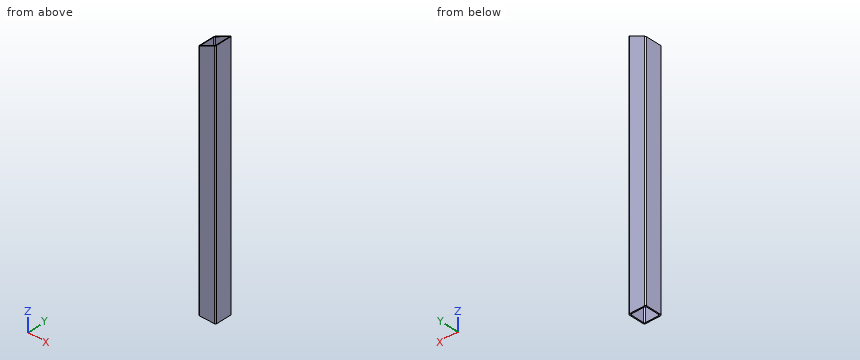
```python
from build123d import *

# Parameters (mm, degrees)
F1_DEPTH      = 723.9
F3_DEPTH      = 50.8
F3_DEPTH_BACK = 50.8


with BuildPart() as f1:
    # F0 (on Top) → F1 (new body)
    with BuildSketch(Plane.XY):
        with BuildLine():
            ThreePointArc((25.4, 22.225), (24.4700640303, 24.4700640303), (22.225, 25.4))
            Line((22.225, 25.4), (-22.225, 25.4))
            ThreePointArc((-22.225, 25.4), (-24.4700640303, 24.4700640303), (-25.4, 22.225))
            Line((-25.4, 22.225), (-25.4, -22.225))
            ThreePointArc((-25.4, -22.225), (-24.4700640303, -24.4700640303), (-22.225, -25.4))
            Line((-22.225, -25.4), (22.225, -25.4))
            ThreePointArc((22.225, -25.4), (24.4700640303, -24.4700640303), (25.4, -22.225))
            Line((25.4, -22.225), (25.4, 22.225))
        make_face()
        with BuildLine():
            Line((-19.05, 22.225), (19.05, 22.225))
            ThreePointArc((19.05, 22.225), (21.2950640303, 21.2950640303), (22.225, 19.05))
            Line((22.225, 19.05), (22.225, -19.05))
            ThreePointArc((22.225, -19.05), (21.2950640303, -21.2950640303), (19.05, -22.225))
            Line((19.05, -22.225), (-19.05, -22.225))
            ThreePointArc((-19.05, -22.225), (-21.2950640303, -21.2950640303), (-22.225, -19.05))
            Line((-22.225, -19.05), (-22.225, 19.05))
            ThreePointArc((-22.225, 19.05), (-21.2950640303, 21.2950640303), (-19.05, 22.225))
        make_face(mode=Mode.SUBTRACT)
    extrude(amount=F1_DEPTH)

    # F2 (on Front) → F3 (cut, two sides)
    with BuildSketch(Plane.XZ) as f3_sk:
        Polygon((-25.4, 699.484362387), (25.4, 723.9), (-25.4, 723.9), align=None)
    extrude(amount=-F3_DEPTH, mode=Mode.SUBTRACT)
    extrude(f3_sk.sketch, amount=F3_DEPTH_BACK, mode=Mode.SUBTRACT)


solid = f1.part
```
Can you work these out from the model? Positions are in its coordinate system, mm. Give positions to 0.01 mm unless a question says otherwise; leave off trailing zeros. Loops run counter-clockwise (first coordinate to the right, second up) from the corner with the lowest first, then second, coordinate; pieces in that order, holes last. Notation, with made-up numbers: M -11.75,-21.75 L 35.25,-21.75 A15 cw 35.25,-17.75 Z; hole C 16,5.5 d7. An arc over 180 degrees is marked long. Use one line per item in the form item = value. Start each with the question number.
(1) I want a section at A-A, the plane y = 7. Write out the boundary of the cut face in (x, z) (3 decimals), and give its area (3 significant figures).
(2) I'm going to push a flat-ended pin straight in: P1, Ø1, axis at x = -20, y = 10, coming from the +Z side. Where does the tip first touch, or does it pass through?
(3) I want a section at C-C, the plane x = 4. Write out the boundary of the cut face in (y, z) (3 decimals).
(4) Please list where these lines run through material, in increasing order: line 1 (Y direction, x = -15, z = 280.5) (3 decimals); line 2 (X direction, y = -20, z = 343.5).
(5) I want a section at B-B, the plane z = 83.5. Write out the boundary of the cut face in (x, y) (3 decimals), and give its area (3 significant figures).
Worked out:
q1.outline = M -25.4,0 L -22.225,0 L -22.225,701.01 L -25.4,699.484 Z; M 22.225,0 L 25.4,0 L 25.4,723.9 L 22.225,722.374 Z
q1.area = 4,520 mm²
q2.P1 = through
q3.outline = M -25.4,0 L -22.225,0 L -22.225,713.615 L -25.4,713.615 Z; M 22.225,0 L 25.4,0 L 25.4,713.615 L 22.225,713.615 Z
q4.line_1 = -25.4 to -22.225, 22.225 to 25.4
q4.line_2 = -25.4 to -22.08, 22.08 to 25.4
q5.outline = M -25.4,-22.225 A3.175 ccw -22.225,-25.4 L 22.225,-25.4 A3.175 ccw 25.4,-22.225 L 25.4,22.225 A3.175 ccw 22.225,25.4 L -22.225,25.4 A3.175 ccw -25.4,22.225 Z; hole M -22.225,-19.05 A3.175 ccw -19.05,-22.225 L 19.05,-22.225 A3.175 ccw 22.225,-19.05 L 22.225,19.05 A3.175 ccw 19.05,22.225 L -19.05,22.225 A3.175 ccw -22.225,19.05 Z
q5.area = 605 mm²
